Check sheet for the modelled part. Datum: model origin and axes. Units: mm. A direction names the side the tool comes from. Round coordinates to 2 decimals unless told otherwise and drop trailing zeros. Order: outer loops, then holes, each group sorted by start corner. A loop starts at its lowest first (then second) coordinate and runs counter-clockwise, first axis right, second up. Notation, with made-up numbers: (19.5, 35) -> (58.5, 35) arc R16 cw to (58.5, 57) -> close; hole circle Ø11 at (36, 31.5). An arc over 180 degrees is marked (long way). Answer in a Markdown table with one row per item.
from build123d import *

# Parameters (mm, degrees)
BOSS_EXTRU_1_DEPTH      = 36
BOSS_EXTRU_2_DEPTH      = 6
BOSS_EXTRU_2_DEPTH_BACK = 48


with BuildPart() as part:
    # Esquisse1 → Boss.-Extru.1 (new body)
    with BuildSketch(Plane.XY):
        Polygon((6.070596481, -169.485418462), (-149.8139762, -79.485418462), (-146.8139762, -74.28926604), (9.070596481, -164.28926604), align=None)
    extrude(amount=BOSS_EXTRU_1_DEPTH)

    # Esquisse3 → Boss.-Extru.2 (add, two sides: drawn at the far end of the back side and taken through both)
    with BuildSketch(Plane(origin=(0, 0, 0), x_dir=(-1, 0, 0), z_dir=(0, 0, -1)).offset(-BOSS_EXTRU_2_DEPTH_BACK)):
        Polygon((32.4986229, -140.28926604), (8.249911594, -154.28926604), (11.249911594, -159.485418462), (35.4986229, -145.485418462), align=None)
        Polygon((68.871689859, -119.28926604), (56.747334206, -126.28926604), (59.747334206, -131.485418462), (71.871689859, -124.485418462), align=None)
        Polygon((80.996045512, -112.28926604), (68.871689859, -119.28926604), (71.871689859, -124.485418462), (83.996045512, -117.485418462), align=None)
        Polygon((129.493468124, -84.28926604), (105.244756818, -98.28926604), (108.244756818, -103.485418462), (132.493468124, -89.485418462), align=None)
    extrude(amount=BOSS_EXTRU_2_DEPTH + BOSS_EXTRU_2_DEPTH_BACK)


solid = part.part
Item 1: Scan lines: line 1 (Z direction, x = -139, y = -81.5); line 2 (X direction, y = -90, z = 18.5); line 3 (Y direction, x = -32, z = 15). Record each from-to range of solid material in increasing order. Write a range as [from, to].
Result sheet:
| item | result |
|---|---|
| line 1 | z = [0, 36] |
| line 2 | x = [-131.6, -119.6] |
| line 3 | y = [-147.51, -140.58] |
Item 2: Set-up check for faces 1 (the flat face through (-34.02, -142.924, -2.958)), 2 (the flat face through (-58.226, -128.851, -2.958)), 3 (the flat face through (-9.73, -156.85, 42.08)): record each of +Z, -Z, +X, -X, +Y, -Y from which the full face is reachable in a straight line by a thin tool's end or side.
Result sheet:
| item | result |
|---|---|
| face 1 | -Z, -X, +Y |
| face 2 | -Z, +X, -Y |
| face 3 | +Z, +X, -Y |
Item 3: Cross-section at A-A (z = 39). Record the boundary of the cut face in (x, y).
Result sheet:
| item | result |
|---|---|
| outline | (-132.49, -89.49) -> (-108.24, -103.49) -> (-105.24, -98.29) -> (-129.49, -84.29) -> close; (-84, -117.49) -> (-59.75, -131.49) -> (-56.75, -126.29) -> (-81, -112.29) -> close; (-35.5, -145.49) -> (-11.25, -159.49) -> (-8.25, -154.29) -> (-32.5, -140.29) -> close |
Item 4: Cross-section at D-D (z = 13). Record the boundary of the cut face in (x, y), and give its area (3 significant figures).
Result sheet:
| item | result |
|---|---|
| outline | (-149.81, -79.49) -> (6.07, -169.49) -> (9.07, -164.29) -> (-146.81, -74.29) -> close |
| area | 1,080 mm^2 |
Item 5: Cross-section at C-C (x = -119.5). Record the boundary of the cut face in (y, z), and give its area (3 significant figures).
Result sheet:
| item | result |
|---|---|
| outline | (-96.99, -6) -> (-90.06, -6) -> (-90.06, 48) -> (-96.99, 48) -> close |
| area | 374 mm^2 |
Item 6: Cross-section at B-B (y = -157). Record the boundary of the cut face in (x, z), and give its area (3 significant figures).
Result sheet:
| item | result |
|---|---|
| outline | (-15.55, -6) -> (-9.81, -6) -> (-9.81, 0) -> (-3.55, 0) -> (-3.55, 36) -> (-9.81, 36) -> (-9.81, 48) -> (-15.55, 48) -> close |
| area | 535 mm^2 |
Item 7: Depth check by flat-ended pin: P1, Ø4.5, axis at x = 0.5, y = -165, coming from the -Z side; P2, Ø6, axis at x = -45.5, y = -135, coming from the +Z side; P3, Ø3, axis at y = -105, z = 34, coming from the +X side. Enter the tip coordinate at first touch or a pass-through.
Result sheet:
| item | result |
|---|---|
| P1 | stops at z = 0 |
| P2 | stops at z = 36 |
| P3 | stops at x = -91.02 |
